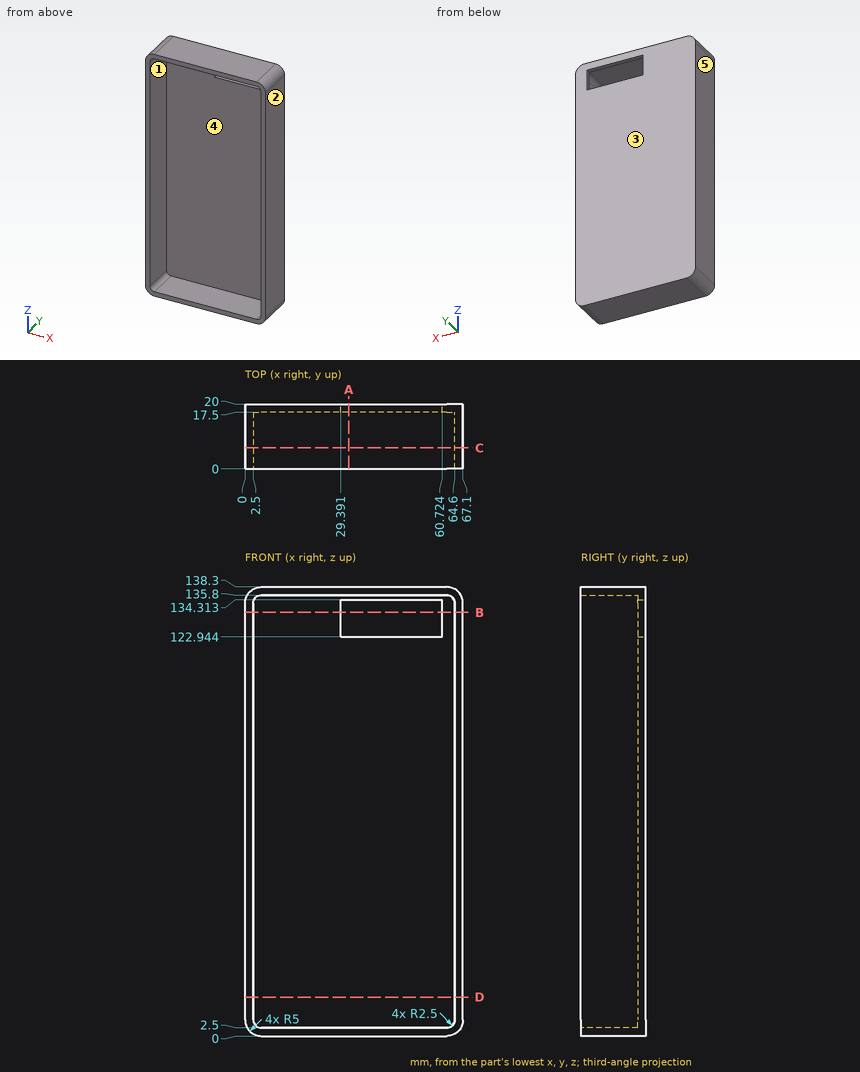
Geometry check sheet. Reference: drawing and pictorial views, mm from the part's lowest x, y, z. A direction names the side the tool comes from. Coordinates: 2 decimals unless noted, no trailing zeros. Loops run counter-clockwise (first coordinate to the right, second up) from the corner with the lowest first, then second, coordinate; pieces in that order, holes last. Notation, with made-up numbers: M 3,36.5 L 21,36.5 A15 cw 21,41.5 Z; hole C 53.25,65.25 d2. An arc over 180 degrees is marked long. One line per item, written item: value.
1. Gauge pin test, flat end, axial feed: P1, Ø4, axis at x = 12.5, z = 89.5, coming from the -Y side. Record the tip position at first contact, or that the pin passes through.
Answers follow:
P1: y = 17.5
2. Mould release check, pull along X, two halves, no side actions. Record for the marked faces 3, 4 and 5: pulls with the +X half, pulls with the -X half, needs draft (parallel to the pull), parting line crosses it, or undercut.
Answers follow:
face 3: needs draft
face 4: undercut
face 5: pulls with the -X half
3. Section check A-A on x = 32. Record the cut outline in (y, z), plus the area to 3 significant figures.
Answers follow:
outline: M 0,0 L 20,0 L 20,122.94 L 17.5,122.94 L 17.5,2.5 L 0,2.5 Z; M 0,135.8 L 17.5,135.8 L 17.5,134.31 L 20,134.31 L 20,138.3 L 0,138.3 Z
area: 405 mm^2
4. Material ranges on line 1 along Z through (x, y) = (34.5, 3.25); line 2 along X through (y, z) = (14.25, 55); line 3 along Y through (x, z) = (62, 121), recorded low to high. Write a range as from..to.
Answers follow:
line 1: 0..2.5, 135.8..138.3
line 2: 0..2.5, 64.6..67.1
line 3: 17.5..20
5. Section check D-D on z = 12. Record the cut outline in (x, y), plus the area to 3 significant figures.
Answers follow:
outline: M 0,0 L 2.5,0 L 2.5,17.5 L 64.6,17.5 L 64.6,0 L 67.1,0 L 67.1,20 L 0,20 Z
area: 255 mm^2
6. Set-up check for the marked faces 1 and 2: record each of +Z, -Z, +X, -X, +Y, -Y from which the full face is reachable in a straight line by a thin tool's end or side.
Answers follow:
face 1: -Y
face 2: +Z, -Z, +X, +Y, -Y
7. Section check B-B on z = 130.5. Record the cut outline in (x, y), plus the area to 3 significant figures.
Answers follow:
outline: M 0,0 L 2.5,0 L 2.5,17.5 L 29.39,17.5 L 29.39,20 L 0,20 Z; M 60.72,17.5 L 64.6,17.5 L 64.6,0 L 67.1,0 L 67.1,20 L 60.72,20 Z
area: 177 mm^2
8. Section check C-C on y = 6.5. Record the cut outline in (x, z).
Answers follow:
outline: M 0,5 A5 ccw 5,0 L 62.1,0 A5 ccw 67.1,5 L 67.1,133.3 A5 ccw 62.1,138.3 L 5,138.3 A5 ccw 0,133.3 Z; hole M 2.5,5 A2.5 ccw 5,2.5 L 62.1,2.5 A2.5 ccw 64.6,5 L 64.6,133.3 A2.5 ccw 62.1,135.8 L 5,135.8 A2.5 ccw 2.5,133.3 Z
